Check sheet for the drawn part. Datum: minimum x, y, z corner. Units: mm. A direction names the side the tool comes from. Give positions to 0.01 mm unless a question says otherwise; leave off trailing zeros. Loops run counter-clockwise (first coordinate to the right, second up) from the corner with the lowest first, then second, coordinate; pieces in that order, holes last. Notation, with made-up numbers: (3, 55) - (37, 55) arc R8 cw to (37, 70) - close; hole circle Ø1 at (48.25, 28). An arc over 180 degrees is marked (long way). Use one line per item in the form item = value.
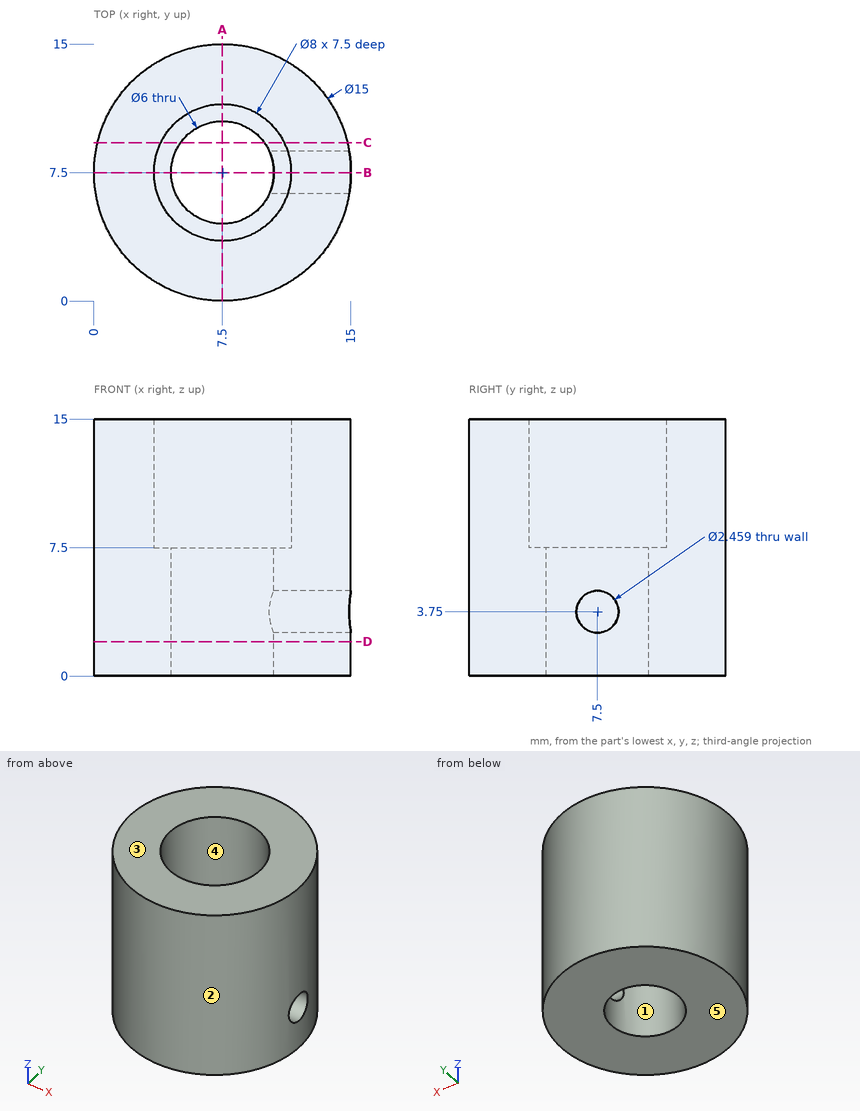
Item 1: Section check A-A on x = 7.5. Record the boundary of the cut face in (y, z).
Answer block:
outline = (0, 0) - (4.5, 0) - (4.5, 7.5) - (3.5, 7.5) - (3.5, 15) - (0, 15) - close; (10.5, 0) - (15, 0) - (15, 15) - (11.5, 15) - (11.5, 7.5) - (10.5, 7.5) - close
Item 2: Section check B-B on y = 7.5. Record the boundary of the cut face in (x, z).
Answer block:
outline = (0, 0) - (4.5, 0) - (4.5, 7.5) - (3.5, 7.5) - (3.5, 15) - (0, 15) - close; (10.5, 0) - (15, 0) - (15, 2.52) - (10.5, 2.52) - close; (10.5, 4.98) - (15, 4.98) - (15, 15) - (11.5, 15) - (11.5, 7.5) - (10.5, 7.5) - close
Item 3: Gauge pin test, flat ends, axial feed: P1, Ø1, axis at x = 4, z = 6, coming from the -Y side; P2, Ø8, axis at y = 2.5, z = 10.5, coming from the +X side; P3, Ø6.5, axis at x = 7.5, y = 7.5, coming from the +Z side. Record the tip position at first contact, or that the pin passes through.
Answer block:
P1 = 0.63
P2 = 14.93
P3 = 7.5
Item 4: Access from +Z, -Z, +X, -X, +Y, -Y to the whole of each face (thin tool, end or side, straight path). Record for the marked faces 4 and 5.
Answer block:
face_4 = +Z
face_5 = -Z, +X, -X, +Y, -Y
Item 5: Section check D-D on z = 2. Record the boundary of the cut face in (x, y).
Answer block:
outline = circle Ø15 at (7.5, 7.5); hole circle Ø6 at (7.5, 7.5)
Item 6: Thickness scan on L1, parallel to Y at x = 7.5, z = 12.5; L2, parallel to Y at x = 7.5, z = 2.5; L3, parallel to X at y = 10.75, z = 8. Record the ranges inside material, lowest first.
Answer block:
L1 = 0 to 3.5, 11.5 to 15
L2 = 0 to 4.5, 10.5 to 15
L3 = 0.74 to 5.17, 9.83 to 14.26
Item 7: Mould release check, pull along X, two halves, no side actions. Record for the marked faces 1, 2 and 3: released by +X, released by -X, zero draft, split by the parting line, or undercut.
Answer block:
face_1 = undercut
face_2 = split by the parting line
face_3 = zero draft
Item 8: Section check C-C on y = 9.25. Record the boundary of the cut face in (x, z).
Answer block:
outline = (0.21, 0) - (5.06, 0) - (5.06, 7.5) - (3.9, 7.5) - (3.9, 15) - (0.21, 15) - close; (9.94, 0) - (14.79, 0) - (14.79, 15) - (11.1, 15) - (11.1, 7.5) - (9.94, 7.5) - close
